Autodesk Fusion 360 part; units mm, degrees
sketch "Boceto1" plane through (0, 0, 0) normal (0, 0, 1) x (1, 0, 0)
  line L0 (0, 0) -> (0, 50)
  line L1 (0, 0) -> (0, -50)
  line L2 (0, 50) -> (58, 50)
  line L3 (58, 50) -> (58, -50)
  line L4 (58, -50) -> (0, -50)
extrude "Extruir1" add sketch "Boceto1" along normal blind 4 makes body 1
sketch "Boceto2" plane through (0, 0, 0) normal (0, 1, 0) x (1, 0, 0)
sketch "Boceto3" plane through (58, 0, 0) normal (1, 0, 0) x (0, 1, 0)
  line L0 (-50, 0) -> (50, 0)
  line L1 (50, 0) -> (50, 4)
  line L2 (50, 4) -> (-50, 4)
  line L3 (-50, 4) -> (-50, 0)
  line L4 (-50, 4) -> (-50, 50)
  line L5 (50, 4) -> (50, 20)
  line L6 (-40, 60) -> (-10, 60)
  line L7 (0, 50) -> (0, 40)
  line L8 (10, 30) -> (40, 30)
  arc A0 (-40, 60) -> (-50, 50) centre (-40, 50) ccw
  arc A1 (0, 50) -> (-10, 60) centre (-10, 50) ccw
  arc A2 (0, 40) -> (10, 30) centre (10, 40) ccw
  arc A3 (50, 20) -> (40, 30) centre (40, 20) ccw
  circle A4 centre (-25, 40) radius 5
  dimension "d8" = 10
  dimension "d9" = 10
extrude "Extruir2" add sketch "Boceto3" against normal blind 4 contours L2 L4 L5 L6 L7 L8 A0 A1 A2 A3 | A4 bodies 1
extrude "Extruir3" cut sketch "Boceto3" against normal blind 15 contours A4 bodies 1
split "Dividir1" by plane through (0, 0, 4) normal (0, 0, 1) bodies 1 makes body 2 at (54, 2.859, 12.7006)
copy_body "CopiarPegarCuerpos1" bodies 2 makes body 3
move_body "Desplazar1" bodies 3 to x (1, 0, 0) y (0, 1, 0) z (0, 0, 1) at (-54, 0, 0)
combine "Combinar1" operation add target body 2 tool bodies 3 1
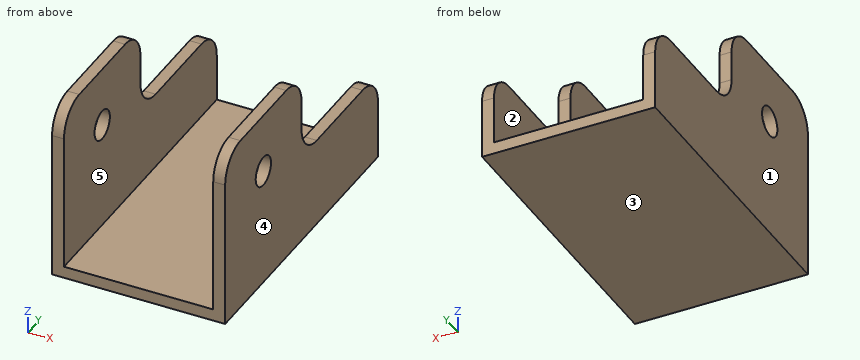
Could you check a few things on this model? Use its own coordinates, in mm. Face numbers are marked on the shaded views. A direction names the side the tool comes from. Round coordinates to 2 decimals unless told otherwise and drop trailing zeros. Write each loop counter-clockwise with the first axis right and the second up, starting at its lowest first coordinate (ties: lowest second). Pieces come first, ordered by that corner, then holes. Notation, with made-up numbers: (49, 6.25) -> (74, 6.25) arc R23 ccw to (74, 43.25) -> close; hole circle Ø8 at (-12, -16). An arc over 180 degrees is marked (long way). Use a Markdown table: item, result.
1. Please list where these lines run through material, in increasing order: probe 1 along X at (y, z) = (13.5, 10); probe 2 along Z at (x, y) = (1.2, -25); probe 3 along Z at (x, y) = (26, 27.5).
Answer key:
| item | result |
|---|---|
| probe 1 | x = 0 to 4, 54 to 58 |
| probe 2 | z = 0 to 35, 45 to 60 |
| probe 3 | z = 0 to 4 |
2. We'd pull the mould along X, two halves only. Please class the marked faces 3, 4 and 5: +X half, -X half, draft (parallel to the pull), parting line (faces both ways), or undercut.
Answer key:
| item | result |
|---|---|
| face 3 | draft |
| face 4 | +X half |
| face 5 | undercut |
3. If we section it at C-C (y = 29): List the corners of the cut face in (x, z) for me, then the cut area to 3 significant figures.
Answer key:
| item | result |
|---|---|
| outline | (0, 0) -> (58, 0) -> (58, 30) -> (54, 30) -> (54, 4) -> (4, 4) -> (4, 30) -> (0, 30) -> close |
| area | 440 mm^2 |
4. If we section it at A-A (y = -25): List the corners of the cut face in (x, z) for me.
Answer key:
| item | result |
|---|---|
| outline | (0, 0) -> (58, 0) -> (58, 35) -> (54, 35) -> (54, 4) -> (4, 4) -> (4, 35) -> (0, 35) -> close; (0, 45) -> (4, 45) -> (4, 60) -> (0, 60) -> close; (54, 45) -> (58, 45) -> (58, 60) -> (54, 60) -> close |
5. For pin 1 Ø4 at (x, y) = (6.5, -16.5) entering from +Z; pin 2 Ø2 at (x, y) = (56, 21.5) entering from +Z; pin 3 Ø3 at (x, z) = (55.5, 45) entering from +Y, each with a flat end and sliding along its axis, tell me the tip position at first contact or that it passes through.
Answer key:
| item | result |
|---|---|
| pin 1 | stops at z = 4 |
| pin 2 | stops at z = 30 |
| pin 3 | stops at y = 0 |
6. Which directions (+Z, -Z, +X, -X, +Y, -Y) give clear straight access to the entire face, cutting with the end or side of a thin tool? Please do the marked faces 1 and 2.
Answer key:
| item | result |
|---|---|
| face 1 | +Z, -Z, -X, +Y, -Y |
| face 2 | +Z, +Y, -Y |
7. If we section it at D-D (x = 8): List the corners of the cut face in (y, z) for me, then the cut area to 3 significant figures.
Answer key:
| item | result |
|---|---|
| outline | (-50, 0) -> (50, 0) -> (50, 4) -> (-50, 4) -> close |
| area | 400 mm^2 |
8. If we section it at B-B (z = 54): List the corners of the cut face in (x, y) for me.
Answer key:
| item | result |
|---|---|
| outline | (0, -49.17) -> (4, -49.17) -> (4, -0.83) -> (0, -0.83) -> close; (54, -49.17) -> (58, -49.17) -> (58, -0.83) -> (54, -0.83) -> close |
